Build history of the part. All positions in model axes, mm. A direction names the side the tool comes from. Give positions to 0.01 mm unless a question says otherwise; leave off trailing zeros. Loops run counter-clockwise (first coordinate to the right, second up) from the corner with the lowest first, then second, coordinate; pieces in that order, holes last.
1) Band-saw the part on A-A on z = 11.5. List the corners of the cut face in (x, y), then the cut area to 3 significant figures.
2) Wall check: line 1 (X direction, y = 7.5, z = 14.5); line 2 (Z direction, x = 14, y = 5.5); line 3 (Y direction, x = 18, z = 1.75). Give the ranges that are in metal, low to high.
3) Band-saw the part on D-D on z = 8.25. List the corners of the cut face in (x, y), then the cut area to 3 significant figures.
4) 3-axis set-ups, long thin cutter, end or side, ignore diameter. For faces 4 (the flat face through (25, 8.268, 8)), 5 (the flat face through (-2, 5.347, 11)), 6 (the flat face through (-2, 2.878, 11)), 7 (the flat face through (-2, 4, 8.955)), 8 (the flat face through (-2, 4, 13.433)): which of +Z, -Z, +X, -X, +Y, -Y reach the whole face in a straight line?
5) Band-saw the part on B-B on x = 34. List the corners of the cut face in (y, z), then the cut area to 3 significant figures.
6) Flat gauge pins, fed straight in: P1, Ø2, axis at y = 4.5, z = 7.5, coming from the -X side; P2, Ø2, axis at x = -2.5, y = 4, coming from the +Z side; P3, Ø1.7, axis at x = -2, z = 10, coming from the +Y side. Where does each tip first touch, or does it go through?
7) Two-plate mould, pull along Z, no slides. Class faces 1 (the flat face through (-2, 4, 12.916)), 2 (the flat face through (25, 4, 17.045)), 3 (the flat face through (0, 4.1, 8.6)): +Z half, -Z half, draft (parallel to the pull), parting line (faces both ways), or undercut.
8) Band-saw the part on C-C on y = 4.5. List the corners of the cut face in (x, z).
```python
from build123d import *

# Parameters (mm, degrees)
F1_DEPTH = 51.562
F2_R     = 3.066051
F3_W     = 3.014619
F3_H     = 4.478862
F3_W_2   = 1.843878
F3_H_2   = 3.103115
F4_DEPTH = 3.3528


with BuildPart() as f1:
    # F0 (on Right) → F1 (new body)
    with BuildSketch(Plane.YZ):
        Polygon((0, 17.045056), (0, 0), (4.706469, 0), (8.268126, 0), (8.268126, 17.045056), (4.706469, 17.045056), align=None)
    extrude(amount=F1_DEPTH)

    # F2
    f2_edges = [f1.edges().sort_by_distance(p)[0] for p in [
        (25.781, 8.268126, 17.045056),
        (25.781, 0, 17.045056),
        (25.781, 8.268126, 0),
        (25.781, 0, 0),
    ]]
    fillet(f2_edges, radius=F2_R)

    # F3 (on Right) → F4 (join)
    with BuildSketch(Plane.YZ):
        with Locations((4.38504, 11.194011)):
            Rectangle(F3_W, F3_H)
        with Locations((4.424905, 11.364611)):
            Rectangle(F3_W_2, F3_H_2, mode=Mode.SUBTRACT)
    extrude(amount=-F4_DEPTH)


solid = f1.part
```
Findings below:
1. outline: (-3.35, 2.88) - (0, 2.88) - (0, 0) - (51.56, 0) - (51.56, 8.27) - (0, 8.27) - (0, 5.89) - (-3.35, 5.89) - (-3.35, 5.35) - (0, 5.35) - (0, 3.5) - (-3.35, 3.5) - close
1. area: 430 mm2
2. line 1: x = 0 to 51.56
2. line 2: z = 0.01 to 17.03
2. line 3: y = 0.3 to 7.97
3. outline: (0, 0) - (51.56, 0) - (51.56, 8.27) - (0, 8.27) - close
3. area: 426 mm2
4. face 4: +Z, -Z, +X, -X, +Y
4. face 5: -X
4. face 6: +Z, -Z, -X, -Y
4. face 7: -Z, -X, +Y, -Y
4. face 8: +Z, -X, +Y, -Y
5. outline: (0, 3.07) arc R3.07 ccw to (3.07, 0) - (5.2, 0) arc R3.07 ccw to (8.27, 3.07) - (8.27, 13.98) arc R3.07 ccw to (5.2, 17.05) - (3.07, 17.05) arc R3.07 ccw to (0, 13.98) - close
5. area: 133 mm2
6. P1: stops at x = 0
6. P2: stops at z = 13.43
6. P3: stops at y = 5.89
7. face 1: undercut
7. face 2: +Z half
7. face 3: draft
8. outline: (-3.35, 8.95) - (0, 8.95) - (0, 0) - (51.56, 0) - (51.56, 17.05) - (0, 17.05) - (0, 13.43) - (-3.35, 13.43) - (-3.35, 12.92) - (0, 12.92) - (0, 9.81) - (-3.35, 9.81) - close
